Geometry check sheet. Reference: drawing and pictorial views, mm from the part's lowest x, y, z. A direction names the side the tool comes from. Give positions to 0.01 mm unless a question says otherwise; leave off trailing zeros. Order: outer loops, then holes, each group sorted by start corner. A loop starts at its lowest first (then second) coordinate and runs counter-clockwise, first axis right, second up.
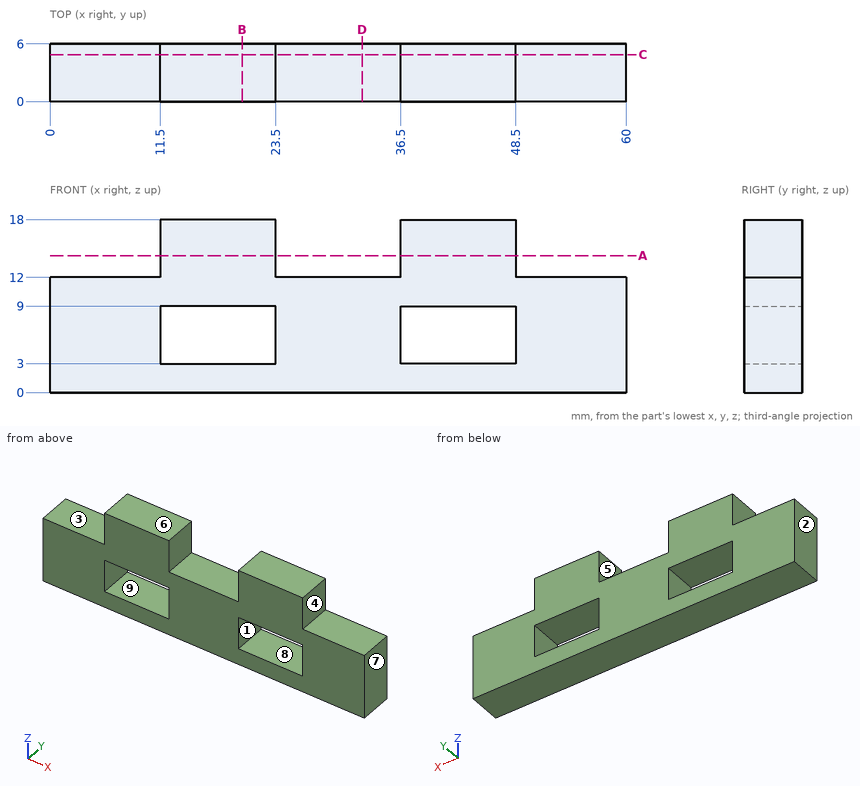
(1) Sectioned sample at D-D (x = 32.5). Enter the section's corners in (y, z), plus the area to 3 significant figures.
(2) Sectioned sample at A-A (z = 14.25). Enter the section's corners in (x, y), plus the area to 3 significant figures.
(3) Sectioned sample at B-B (x = 20). Enter the section's corners in (y, z).
(4) Release check for a two-part mould opening along Z. For the marked faces 6, 7, 8 and 9 record: released by +Z, released by -Z, zero draft, split by the parting line, or undercut.
(5) Thickness scan on L1, parallel to X at y = 2.05, z = 8.75; L2, parallel to X at y = 0.7, z = 14.25; L3, parallel to Z at x = 47, y = 4.35. Record the ranges inside material, lowest first.
(6) Tool access check on the marked faces 1, 2, 3, 4 and 5. Record the directions out of +Z, -Z, +X, -X, +Y, -Y that give a thin tool (end or side, any length) a straight path to the whole face; none if there is none.
(7) Go/stop test with flat-tipped pins: P1, Ø1.8, axis at x = 8, y = 4.5, coming from the +Z side; P2, Ø3, axis at y = 4, z = 14.5, coming from the +X side. Record where each tip stops, or that it passes through.
(8) Sectioned sample at C-C (y = 4.9). Enter the section's corners in (x, z).
Values follow:
1. outline: (0, 0) - (6, 0) - (6, 12) - (0, 12) - close
1. area: 72.0 mm2
2. outline: (11.5, 0) - (23.5, 0) - (23.5, 6) - (11.5, 6) - close; (36.5, 0) - (48.5, 0) - (48.5, 6) - (36.5, 6) - close
2. area: 144 mm2
3. outline: (0, 0) - (6, 0) - (6, 3) - (0, 3) - close; (0, 9) - (6, 9) - (6, 18) - (0, 18) - close
4. face 6: released by +Z
4. face 7: zero draft
4. face 8: undercut
4. face 9: undercut
5. L1: x = 0 to 11.5, 23.5 to 36.5, 48.5 to 60
5. L2: x = 11.5 to 23.5, 36.5 to 48.5
5. L3: z = 0 to 3, 9 to 18
6. face 1: +Y, -Y
6. face 2: +Z, -Z, -X, +Y, -Y
6. face 3: +Z, -X, +Y, -Y
6. face 4: +Z, +X, +Y, -Y
6. face 5: +Z, +Y, -Y
7. P1: stops at z = 12
7. P2: stops at x = 48.5
8. outline: (0, 0) - (60, 0) - (60, 12) - (48.5, 12) - (48.5, 18) - (36.5, 18) - (36.5, 12) - (23.5, 12) - (23.5, 18) - (11.5, 18) - (11.5, 12) - (0, 12) - close; hole (11.5, 3) - (23.5, 3) - (23.5, 9) - (11.5, 9) - close; hole (36.5, 3) - (48.5, 3) - (48.5, 9) - (36.5, 9) - close
